Check sheet for the modelled part. Datum: model origin and axes. Units: mm. Face numbers are marked on the shaded views. A direction names the side the tool comes from. Round coordinates to 2 decimals unless told otherwise and drop trailing zeros. Order: outer loops, then holes, each group sorted by start corner. A loop starts at its lowest first (then second) coordinate and runs counter-clockwise, first axis right, second up.
(1) Sectioned sample at C-C, the plane z = -36. Enter the section's corners in (x, y), and give its area (3 significant figures).
(2) Sectioned sample at A-A, the plane z = -163.83. Enter the section's corners in (x, y).
(3) Sectioned sample at B-B, the plane y = 6. Count the separate pieces of the cut face and the enclosed holes in it, and give its area (3 significant figures).
(4) Tool access check on the marked faces 5, 6, 7 and 8. Record the directions out of +Z, -Z, +X, -X, +Y, -Y that give a thin tool (end or side, any length) a straight path to the whole face; none if there is none.
(5) Mould release check, pull along Z, two halves, no side actions. Record for the marked faces 1, 2, 3 and 4: released by +Z, released by -Z, zero draft, split by the parting line, or undercut.
(6) Thickness scan on probe 1 along X at (y, z) = (3.25, 0); probe 2 along Z at (x, y) = (15, 23); probe 3 along X at (y, z) = (11.5, -120). Record the ranges inside material, lowest first.
(7) Depth check by flat-ended pin: pin 1 (9 mm diameter, centred on x = 3, y = 19, fed in from +Z); pin 2 (10 mm diameter, centred on x = 14, z = -98, fed in from +Y); pin 3 (3.5 mm diameter, centred on x = -15.494, z = 0, fed in from -Y); pin 4 (1.5 mm diameter, centred on x = 8.5, y = 34.5, fed in from +Z). Enter the tip coordinate at first touch or a pass-through.
Autodesk Inventor part; units mm, degrees
ref_plane "YZ Plane" through (0, 0, 0) normal (1, 0, 0) x (0, 1, 0)
ref_plane "XZ Plane" through (0, 0, 0) normal (0, 1, 0) x (-1, 0, 0)
ref_plane "XY Plane" through (0, 0, 0) normal (0, 0, 1) x (1, 0, 0)
sketch "Sketch1" plane through (0, 0, 0) normal (0, 1, 0) x (-1, 0, 0)
  circle A0 centre (0, 0) radius 22.86
  line L0 (14.5416, -26.67) -> (-16.51, -26.67)
  line L1 (-20.32, -15.24) -> (-20.32, -55.88)
  line L2 (-13.6865, -63.5) -> (16.51, -63.5)
  line L3 (20.32, -55.88) -> (20.32, -15.24)
  line L4 (16.51, -67.31) -> (-16.51, -67.31)
  line L5 (-20.32, -59.69) -> (-20.32, -100.33)
  line L6 (-16.51, -104.14) -> (13.9515, -104.14)
  line L7 (20.32, -100.33) -> (20.32, -59.69)
  line L8 (13.9515, -107.95) -> (-16.51, -107.95)
  line L9 (-20.32, -104.14) -> (-20.32, -144.78)
  line L10 (20.32, -144.78) -> (20.32, -104.14)
  line L11 (20.32, -15.24) -> (20.32, -10.4727)
  circle A1 centre (0, -163.83) radius 6.35
  line L12 (-20.32, -15.24) -> (-20.32, -10.4727)
  line L13 (20.32, -55.88) -> (20.32, -59.69)
  line L14 (20.32, -100.33) -> (20.32, -104.14)
  line L15 (-20.32, -55.88) -> (-20.32, -59.69)
  line L16 (-20.32, -100.33) -> (-20.32, -104.14)
  line L17 (20.32, -144.78) -> (20.32, -148.59)
  line L18 (-20.32, -144.78) -> (-20.32, -148.59)
  line L19 (20.32, -148.59) -> (8.7779, -160.1321)
  line L20 (-20.32, -148.59) -> (-8.7779, -160.1321)
  line L21 (16.51, -30.1719) -> (16.51, -63.5)
  line L22 (-16.51, -26.67) -> (-16.51, -60.9418)
  line L23 (16.51, -67.31) -> (16.51, -101.2863)
  line L24 (-16.51, -67.31) -> (-16.51, -104.14)
  line L25 (16.51, -110.8037) -> (16.51, -144.78)
  line L26 (-16.51, -141.9263) -> (-16.51, -107.95)
  arc A2 (-8.7779, -160.1321) -> (8.7779, -160.1321) centre (0, -163.83) ccw
  line L27 (14.5416, -26.67) -> (-16.51, -60.9418)
  line L28 (16.9388, -26.8614) -> (16.51, -27.3347)
  line L29 (17.3651, -29.2282) -> (-13.6865, -63.5)
  line L30 (-13.9515, -67.31) -> (16.51, -101.2863)
  line L31 (-16.51, -70.1637) -> (13.9515, -104.14)
  line L32 (13.9515, -107.95) -> (-16.51, -141.9263)
  line L33 (16.51, -110.8037) -> (-13.9515, -144.78)
  line L34 (-19.0685, -144.78) -> (-16.51, -144.78)
  line L35 (-13.9515, -144.78) -> (16.51, -144.78)
  dimension "d0" = 45.72
  dimension "d2" = 26.67
  dimension "d3" = 36.83
  dimension "d5" = 20.32
  dimension "d6" = 3.81
  dimension "d7" = 40.64
  dimension "d8" = 3.81
  dimension "d10" = 12.7
  dimension "d11" = 3.81
  dimension "d12" = 3.81
  dimension "d13" = 135
  dimension "d14" = 3.81
  dimension "d15" = 3.81
  dimension "d16" = 3.81
  dimension "d17" = 36.83
  dimension "d19" = 94.2927
  dimension "d20" = 62.8618
  dimension "d21" = 123.0295
  dimension "d22" = 94.2927
  dimension "d23" = 91.5986
  dimension "d24" = 62.8618
  dimension "d25" = 3.81
  dimension "d26" = 36.83
  dimension "d27" = 65.5559
  dimension "d28" = 60.1677
  dimension "d29" = 19.05
  dimension "d32" = 1.905
  dimension "d37" = 42.178
  dimension "d38" = 138.122
  dimension "d39" = 138.122
  dimension "d40" = 118.11
  dimension "d41" = 36.83
  dimension "d42" = 0
  dimension "d43" = 3.81
  dimension "d44" = 3.81
  dimension "d45" = 86.2593
  dimension "d46" = 55.3203
  dimension "d47" = 3.3812
  dimension "d48" = 11.5421
  dimension "d49" = 36.83
  dimension "d50" = 119.4374
  dimension "d51" = 119.4374
  dimension "d52" = 20.32
extrude "Extrusion1" add sketch "Sketch1" along normal blind 40.64
sketch "Sketch2" plane through (0, 40.64, 0) normal (0, 1, 0) x (1, 0, 0)
  circle A0 centre (0, 0) radius 18.415
  dimension "d55" = 36.83
extrude "Extrusion2" cut sketch "Sketch2" against normal blind 36.322
sketch "Sketch3" plane through (0, 4.318, 0) normal (0, 1, 0) x (1, 0, 0)
  circle A0 centre (0, -6.985) radius 6.096
  line L0 (0, 0) -> (0, -18.9723)
  arc A1 (-20.32, 10.4727) -> (20.32, 10.4727) centre (0, 0) ccw
  line L1 (-15.494, 0) -> (15.494, 0)
  circle A2 centre (-15.494, 0) radius 1.9939
  circle A3 centre (15.494, 0) radius 1.9939
  point P0 (0, -22.86)
  dimension "d58" = 6.985
  dimension "d59" = 12.192
  dimension "d61" = 3.9878
  dimension "d62" = 30.988
  dimension "d63" = 15.494
  dimension "d65" = 18.9722
extrude "Extrusion3" cut sketch "Sketch3" against normal blind 36.322
properties part number "leg 2.0"
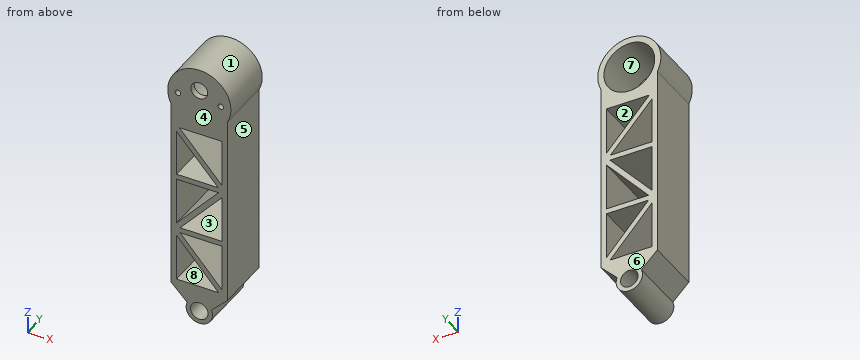
Derived:
1. outline: (-20.32, 0) - (-16.51, 0) - (-16.51, 40.64) - (-20.32, 40.64) - close; (-11.23, 0) - (-6.09, 0) - (-6.09, 40.64) - (-11.23, 40.64) - close; (16.51, 0) - (20.32, 0) - (20.32, 40.64) - (16.51, 40.64) - close
1. area: 519 mm2
2. outline: (-9.53, 0) - (-6.35, 0) - (-6.35, 40.64) - (-9.53, 40.64) - close; (6.35, 0) - (9.53, 0) - (9.53, 40.64) - (6.35, 40.64) - close
3. separate pieces: 1
3. enclosed holes: 8
3. area: 3,150 mm2
4. face 5: -Z, +X, +Y, -Y
4. face 6: +Z, -Z, +X, -X, +Y
4. face 7: +Y
4. face 8: +Y, -Y
5. face 1: split by the parting line
5. face 2: undercut
5. face 3: undercut
5. face 4: zero draft
6. probe 1: x = -22.86 to -17.49, -13.5 to 13.5, 17.49 to 22.86
6. probe 2: z = -153.91 to -140.24, -107.95 to -104.14, -71.85 to -59.28, -26.67 to -10.68, 10.68 to 17.25
6. probe 3: x = -20.32 to -16.51, -8.27 to -3.15, 16.51 to 20.32
7. pin 1: stops at z = 22.86
7. pin 2: stops at y = 40.64
7. pin 3: passes through
7. pin 4: stops at z = 21.51
